Here's the drawing with two shaded views (mm, measured from the low corner). I have some questions. Round coordinates to 2 decimals unless told otherwise and drop trailing zeros. Order: outer loops, then holes, each group sorted by start corner. A loop starts at its lowest first (then second) coordinate and runs counter-clockwise, first axis right, second up.
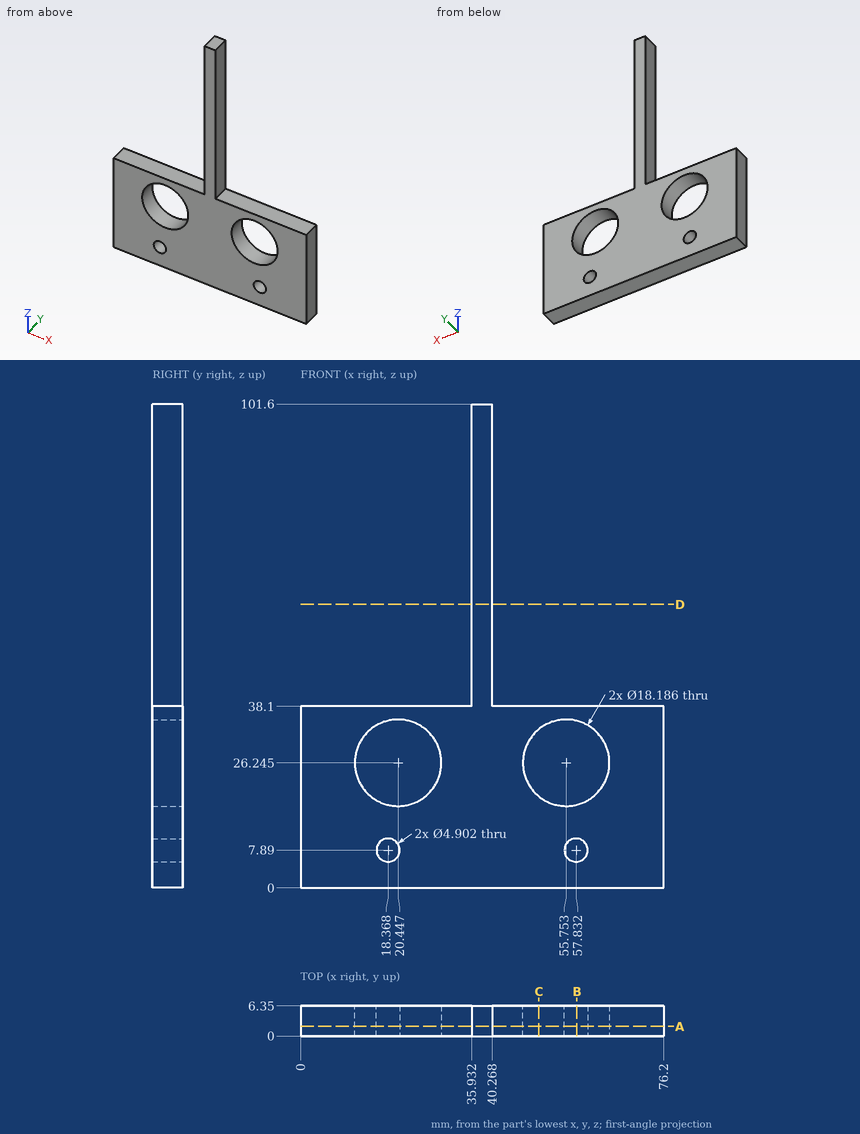
1. I need wall thicknesses on probe 1 along Z at (x, y) = (19.5, 5.5) (1 decimal); probe 2 along X at (y, z) = (1.25, 32) (1 decimal); probe 3 along X at (y, z) = (6.25, 57). Which ranges of each line are inside material? Lowest first, please.
Evaluation:
probe 1: z = 0 to 5.7, 10.1 to 17.2, 35.3 to 38.1
probe 2: x = 0 to 13.4, 27.5 to 48.7, 62.8 to 76.2
probe 3: x = 35.93 to 40.27
2. If we section it at A-A, the plane y = 2: Write out the boundary of the cut face in (x, z) (1 decimal).
Evaluation:
outline: (0, 0) - (76.2, 0) - (76.2, 38.1) - (40.3, 38.1) - (40.3, 101.6) - (35.9, 101.6) - (35.9, 38.1) - (0, 38.1) - close; hole circle Ø18.2 at (20.4, 26.2); hole circle Ø4.9 at (18.4, 7.9); hole circle Ø18.2 at (55.8, 26.2); hole circle Ø4.9 at (57.8, 7.9)
3. If we section it at C-C, the plane x = 50: Write out the boundary of the cut face in (y, z).
Evaluation:
outline: (0, 0) - (6.35, 0) - (6.35, 19.2) - (0, 19.2) - close; (0, 33.29) - (6.35, 33.29) - (6.35, 38.1) - (0, 38.1) - close
4. If we section it at B-B, the plane x = 58: State how many separate pieces and enclosed holes the cut face has.
Evaluation:
separate pieces: 3
enclosed holes: 0
5. If we section it at D-D, the plane z = 59.5: Write out the boundary of the cut face in (x, y).
Evaluation:
outline: (35.93, 0) - (40.27, 0) - (40.27, 6.35) - (35.93, 6.35) - close
6. I'm going to push flat-ended pins straight in: P1, Ø1, axis at y = 4, z = 48.5, coming from the -X side; P2, Ø6.5, axis at x = 57.83, z = 7.89, coming from the -Y side; P3, Ø2, axis at x = 18, y = 4, coming from the +Z side; P4, Ø1.9, axis at y = 4.5, z = 83.5, coming from the +X side. Where does each tip first touch, or does it pass through?
Evaluation:
P1: stops at x = 35.93
P2: stops at y = 0
P3: stops at z = 38.1
P4: stops at x = 40.27
